Part model, mm, in its own coordinate system. A direction names the side the tool comes from. Coordinates: 2 decimals unless noted, no trailing zeros. Loops run counter-clockwise (first coordinate to the right, second up) from the corner with the lowest first, then second, coordinate; pieces in that order, holes last. Notation, with made-up numbers: (66.25, 19) - (124.25, 19) arc R15 ccw to (124.25, 36) - close; hole circle Ø1 at (73.5, 25.5). An arc over 180 degrees is marked (long way). Use a Markdown table: item, result. Add a question column.
1. Band-saw the part on D-D, the plane x = -30.5. Give the cut face in (y, z).
2. Pull direction Y, two halves, no side cores. Call faces 3 (the cylindrical face through (72, -68.7, 2.5)), 4 (the flat face through (-38.637, -25.833, 2.465)), 5 (the flat face through (7, -20, 0)), 6 (the cylindrical face through (-59.111, -63.705, 2.465)): pulls with the +Y half, pulls with the -Y half, needs draft (parallel to the pull), parting line crosses it, or undercut.
3. Band-saw the part on C-C, the plane y = -26. Give the cut face in (x, z), plus the area to 3 significant figures.
4. Band-saw the part on A-A, the plane y = 0. Give the cut face in (x, z), plus the area to 3 significant figures.
5. Wall check: probe 1 along Y at (x, z) = (0, 2); probe 2 along X at (y, z) = (-15, 2.2); probe 3 along X at (y, z) = (-53, 1.4). Give the ranges that are in metal, low to high. Write a range as [from, to].
6. Band-saw the part on B-B, the plane z = 2.9. Give the cut face in (x, y), plus the area to 3 significant figures.
7. Drop flat-ended pins along their axis: pin 1 (6 mm diameter, centred on x = -30.5, y = -19, fed in from -Z); pin 2 (3.5 mm diameter, centred on x = -61.97, y = -64.61, fed in from +Z); pin 3 (3 mm diameter, centred on y = -24, z = 1, fed in from +X); pin 4 (2 mm diameter, centred on x = -15, z = 1, fed in from +Y). Give the stop position or say it passes through.
8. 3-axis set-ups, long thin cutter, end or side, ignore diameter. For faces 1 (the cylindrical face through (-68.735, -71.973, 2.465)), 2 (the flat face through (-26.846, -42.432, 2.465)): which of +Z, -Z, +X, -X, +Y, -Y reach the whole face in a straight line?
from build123d import *

# Parameters (mm, degrees)
SKETCH1_R           = 3
BOSS_EXTRUDE2_DEPTH = 5


with BuildPart() as part:
    # Sketch1 → Boss-Extrude2 (new body)
    with BuildSketch(Plane.XY):
        with BuildLine():
            Line((0.29412641, -14.13907669), (-54.75624353, -71.528460831))
            ThreePointArc((-54.75624353, -71.528460831), (-68.895320221, -71.822587241), (-69.18944663, -57.68351055))
            Line((-69.18944663, -57.68351055), (-7.21660155, 6.92247514))
            ThreePointArc((-7.21660155, 6.92247514), (-0.207978779, 9.997837007), (6.92247514, 7.21660155))
            Line((6.92247514, 7.21660155), (71.525492216, -54.753395907))
            ThreePointArc((71.525492216, -54.753395907), (71.819618625, -68.892472597), (57.680541935, -69.186599007))
            Line((57.680541935, -69.186599007), (0.29412641, -14.13907669))
        make_face()
        with Locations((-61.97284508, -64.605985691)):
            Circle(SKETCH1_R, mode=Mode.SUBTRACT)
        with Locations((64.603017075, -61.969997457)):
            Circle(SKETCH1_R, mode=Mode.SUBTRACT)
        Circle(SKETCH1_R, mode=Mode.SUBTRACT)
    extrude(amount=BOSS_EXTRUDE2_DEPTH)


solid = part.part
Geometry check:
| question | item | result |
|---|---|---|
| 1 | outline | (-46.24, 0) - (-17.35, 0) - (-17.35, 5) - (-46.24, 5) - close |
| 2 | face 3 | parting line crosses it |
| 2 | face 4 | pulls with the +Y half |
| 2 | face 5 | needs draft |
| 2 | face 6 | undercut |
| 3 | outline | (-38.8, 0) - (-11.08, 0) - (-11.08, 5) - (-38.8, 5) - close; (12.66, 0) - (41.55, 0) - (41.55, 5) - (12.66, 5) - close |
| 3 | area | 283 mm^2 |
| 4 | outline | (-13.86, 0) - (-3, 0) - (-3, 5) - (-13.86, 5) - close; (3, 0) - (14.45, 0) - (14.45, 5) - (3, 5) - close |
| 4 | area | 112 mm^2 |
| 5 | probe 1 | y = [-14.45, -3], [3, 10] |
| 5 | probe 2 | x = [-28.25, -0.53], [1.19, 30.08] |
| 5 | probe 3 | x = [-64.7, -36.98], [40.81, 69.7] |
| 6 | outline | (-69.19, -57.68) arc R10 ccw to (-54.76, -71.53) - (0.29, -14.14) - (57.68, -69.19) arc R10 ccw to (71.53, -54.75) - (6.92, 7.22) arc R10 ccw to (-7.22, 6.92) - close; hole circle Ø6 at (-61.97, -64.61); hole circle Ø6 at (0, 0); hole circle Ø6 at (64.6, -61.97) |
| 6 | area | 3,790 mm^2 |
| 7 | pin 1 | stops at z = 0 |
| 7 | pin 2 | passes through |
| 7 | pin 3 | stops at x = 41.03 |
| 7 | pin 4 | stops at y = -0.15 |
| 8 | face 1 | +Z, -Z |
| 8 | face 2 | +Z, -Z, -Y |
